Check sheet for the drawn part. Datum: minimum x, y, z corner. Units: mm. A direction names the side the tool comes from. Coordinates: 2 decimals unless noted, no trailing zeros. Order: outer loops, then holes, each group sorted by start corner. A loop starts at its lowest first (then second) coordinate and runs counter-clockwise, first axis right, second up.
1. Set-up check for the marked faces 1, 2, 3 and 4: record each of +Z, -Z, +X, -X, +Y, -Y from which the full face is reachable in a straight line by a thin tool's end or side.
2. Cross-section at C-C (y = 23). Enter the section's corners in (x, z).
3. Cross-section at B-B (z = 5.75). Enter the section's corners in (x, y) (3 decimals).
4. Cross-section at A-A (y = 15). Enter the section's corners in (x, z) (3 decimals).
5. Cross-section at D-D (x = 35.5). Enter the section's corners in (y, z).
6. Draft check along X on the marked faces 5, 6, 7 and 8. Enter one of: released by +X, released by -X, zero draft, split by the parting line, or undercut.
7. Thickness scan on line 1 (X direction, y = 7.5, z = 1.75) (3 decimals); line 2 (X direction, y = 20.5, z = 2); line 3 (Y direction, x = 9, z = 4.75). Record the ranges inside material, lowest first.
8. Gauge pin test, flat ends, axial feed: pin 1 Ø2 at (x, z) = (48, 5.5) entering from +Y; pin 2 Ø1.9 at (y, z) = (14, 4.5) entering from -X. Record the tip position at first contact, or that the pin passes through.
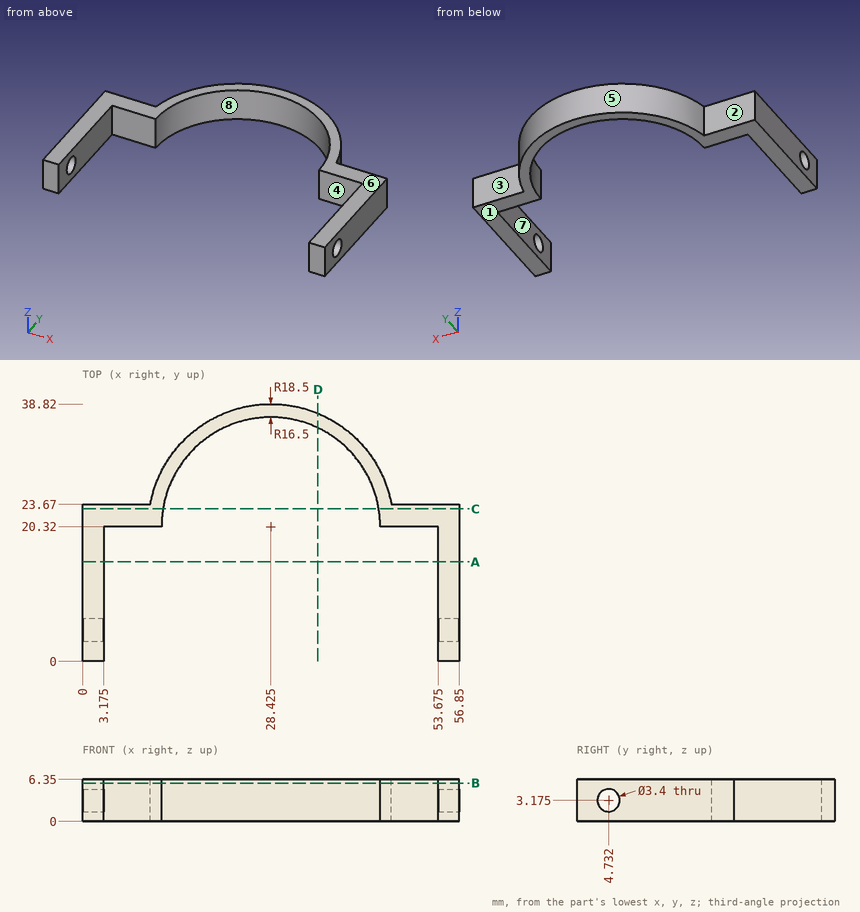
Data:
1. face 1: -Z, +X, -X, +Y, -Y
1. face 2: +Z, -Z, -X, +Y
1. face 3: +Z, -Z, +X, +Y
1. face 4: +Z, -Z, -Y
2. outline: (0, 0) - (12.14, 0) - (12.14, 6.35) - (0, 6.35) - close; (44.71, 0) - (56.85, 0) - (56.85, 6.35) - (44.71, 6.35) - close
3. outline: (0, 0) - (3.175, 0) - (3.175, 20.32) - (11.925, 20.32) arc R16.5 cw to (44.925, 20.32) - (53.675, 20.32) - (53.675, 0) - (56.85, 0) - (56.85, 23.67) - (46.619, 23.67) arc R18.5 ccw to (10.231, 23.67) - (0, 23.67) - close
4. outline: (0, 0) - (3.175, 0) - (3.175, 6.35) - (0, 6.35) - close; (53.675, 0) - (56.85, 0) - (56.85, 6.35) - (53.675, 6.35) - close
5. outline: (35.23, 0) - (37.41, 0) - (37.41, 6.35) - (35.23, 6.35) - close
6. face 5: split by the parting line
6. face 6: zero draft
6. face 7: undercut
6. face 8: undercut
7. line 1: x = 0 to 3.175, 53.675 to 56.85
7. line 2: x = 0 to 11.93, 44.92 to 56.85
7. line 3: y = 20.32 to 23.67
8. pin 1: stops at y = 23.67
8. pin 2: stops at x = 0
